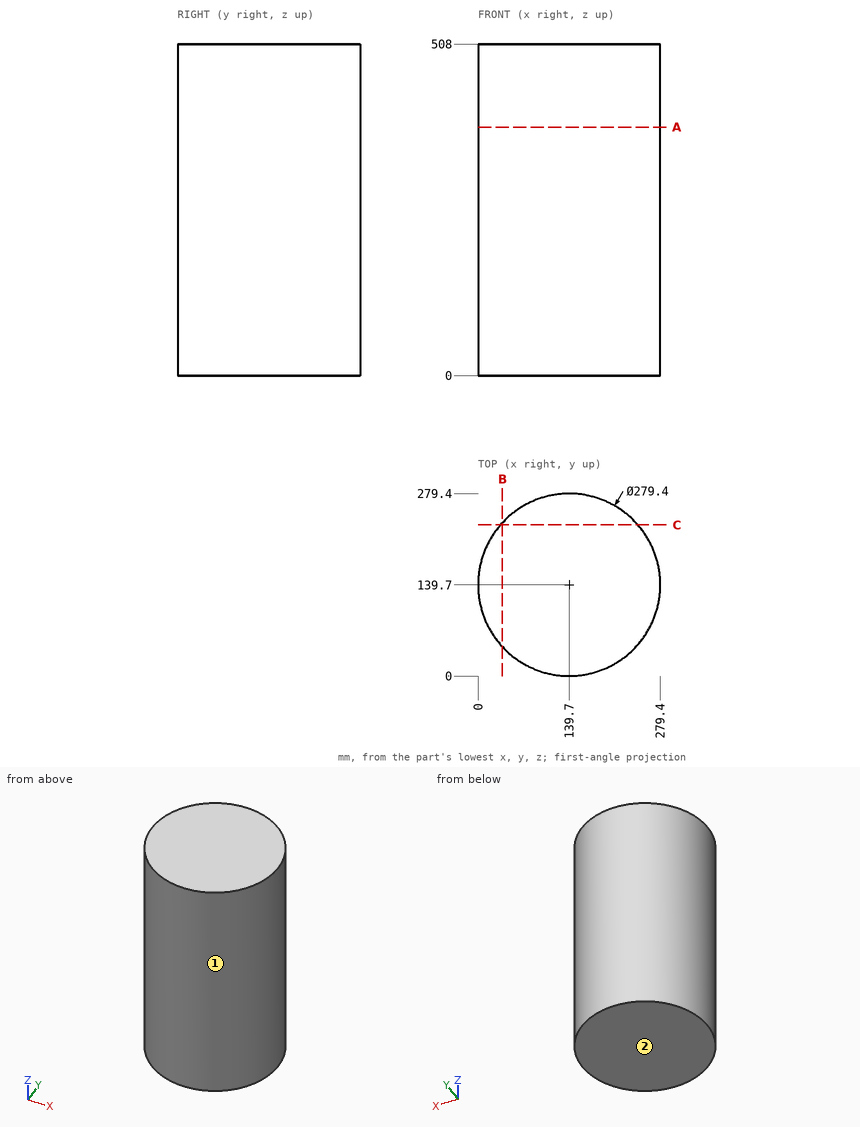
Job drawing, mm, ordinate dimensions from the low corner. One solid piece. Round coordinates to 2 decimals unless told otherwise and drop trailing zeros. Loops run counter-clockwise (first coordinate to the right, second up) from the corner with the lowest first, then second, coordinate; pieces in that order, holes last.
(1) Wall check: line 1 along X through (y, z) = (135.5, 395.5); line 2 along Y through (x, z) = (136, 264); line 3 along Y through (x, z) = (142.5, 190). Give the ranges that are in metal, low to high.
(2) Two-plate mould, pull along Y, no slides. Class the marked faces 1 and 2: +Y half, -Y half, draft (parallel to the pull), parting line (faces both ways), or undercut.
(3) Cut at B-B (x = 37.5). Give the cut face in (y, z), plus the area to 3 significant figures.
(4) Cut at C-C (y = 231.5). Give the cut face in (x, z), plus the area to 3 significant figures.
(5) Cut at A-A (z = 380.5). Give the cut face in (x, y), plus the area to 3 significant figures.
(6) Drop flat-ended pins along their axis: pin 1 (8 mm diameter, centred on x = 203, z = 219.5, fed in from -Y); pin 2 (5 mm diameter, centred on x = 218, z = 346, fed in from -Y); pin 3 (3 mm diameter, centred on y = 230, z = 363.5, fed in from +X). Give the stop position or say it passes through.
Findings below:
1. line 1: x = 0.06 to 279.34
1. line 2: y = 0.05 to 279.35
1. line 3: y = 0.03 to 279.37
2. face 1: parting line
2. face 2: draft
3. outline: (44.46, 0) - (234.94, 0) - (234.94, 508) - (44.46, 508) - close
3. area: 96,800 mm2
4. outline: (34.4, 0) - (245, 0) - (245, 508) - (34.4, 508) - close
4. area: 107,000 mm2
5. outline: circle Ø279.4 at (139.7, 139.7)
5. area: 61,300 mm2
6. pin 1: stops at y = 13.21
6. pin 2: stops at y = 22.35
6. pin 3: stops at x = 247.55
